Geometry: final body of the model. Coordinates: model frame, mm. Give positions to 0.01 mm unless a question says otherwise; leave off trailing zeros. Write each loop counter-clockwise with the first axis right and the second up, starting at its lowest first coordinate (ties: lowest second). Pieces come first, ordered by that corner, then holes. Notation, with made-up numbers: M 18,71.25 L 60,71.25 A6 cw 60,81.25 Z; hole C 49,-35 d3. An arc over 180 degrees is marked long. Use a Markdown table: item, result. Add a question column.
1) Line query: line 1 (X direction, y = 10, z = 49.5); line 2 (Z direction, x = 0.9, y = 12.7) (3 decimals). Output: solid intervals per line, ascending.
2) Section A-A on x = 6.5. Return the cut outline in (y, z), then the cut area to 3 significant figures.
3) Pin query (flat end, axial travel): pin 1 (6.5 mm diameter, centred on x = 8, z = 173, fed in from -Y). Return the tip coordinate at first contact, or that it passes through.
4) Section C-C on z = 19. Return the cut outline in (x, y), then the cut area to 3 significant figures.
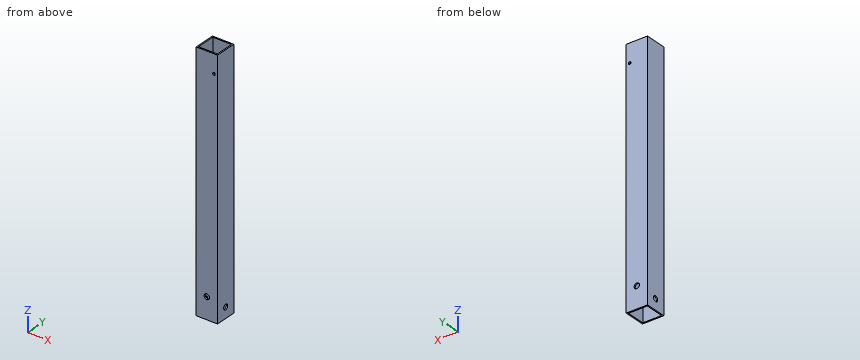
Autodesk Inventor part; units mm, degrees
ref_plane "YZ Plane" through (0, 0, 0) normal (1, 0, 0) x (0, 1, 0)
ref_plane "XZ Plane" through (0, 0, 0) normal (0, 1, 0) x (-1, 0, 0)
ref_plane "XY Plane" through (0, 0, 0) normal (0, 0, 1) x (1, 0, 0)
sketch "Sketch1" plane through (0, 0, 0) normal (0, 0, 1) x (1, 0, 0)
  line L0 (0, 0) -> (25.4, 0)
  line L1 (25.4, 0) -> (25.4, 25.4)
  line L2 (25.4, 25.4) -> (0, 25.4)
  line L3 (0, 25.4) -> (0, 0)
  line L4 (1.5875, 1.5875) -> (23.8125, 1.5875)
  line L5 (23.8125, 1.5875) -> (23.8125, 23.8125)
  line L6 (23.8125, 23.8125) -> (1.5875, 23.8125)
  line L7 (1.5875, 23.8125) -> (1.5875, 1.5875)
  dimension "d0" = 25.4
  dimension "d1" = 25.4
  dimension "d2" = 1.5875
  dimension "d3" = 1.5875
  dimension "d4" = 1.5875
  dimension "d5" = 1.5875
extrude "Extrusion1" add sketch "Sketch1" along normal blind 294.894
sketch "Sketch2" plane through (0, 0, 0) normal (0, -1, 0) x (1, 0, 0)
  line L0 (0, 294.894) -> (25.4, 294.894)
  point P0 (21.1377, 272.796)
  dimension "d15" = 22.098
hole "Hole1" at (21.1377, 0, 272.796) direction (0, 1, 0) diameter 2.9972 end through all
sketch "Sketch3" plane through (0, 0, 0) normal (-1, 0, 0) x (0, 0, 1)
  line L0 (0, 25.4) -> (0, 0)
  line L1 (0, 25.4) -> (294.894, 25.4)
  point P0 (12.7, 12.7)
  dimension "d16" = 12.7
  dimension "d17" = 12.7
hole "Hole2" at (0, 12.7, 12.7) direction (1, 0, 0) diameter 6.35 end through all
sketch "Sketch4" plane through (0, 0, 0) normal (0, -1, 0) x (1, 0, 0)
  line L0 (0, 0) -> (25.4, 0)
  line L1 (0, 0) -> (0, 294.894)
  point P0 (12.7, 25.4)
  dimension "d25" = 25.4
  dimension "d26" = 12.7
hole "Hole3" at (12.7, 0, 25.4) direction (0, 1, 0) diameter 6.35 end through all
properties part number "SwitchBarSupport" material "Aluminum 6061"
Found:
| question | item | result |
|---|---|---|
| 1 | line 1 | 0 to 1.59, 23.81 to 25.4 |
| 1 | line 2 | 0 to 9.525, 15.875 to 294.894 |
| 2 | outline | M 0,0 L 1.59,0 L 1.59,294.89 L 0,294.89 Z; M 23.81,0 L 25.4,0 L 25.4,294.89 L 23.81,294.89 Z |
| 2 | area | 936 mm² |
| 3 | pin 1 | y = 0 |
| 4 | outline | M 0,0 L 25.4,0 L 25.4,25.4 L 0,25.4 Z; hole M 1.59,1.59 L 23.81,1.59 L 23.81,23.81 L 1.59,23.81 Z |
| 4 | area | 151 mm² |
